The listing builds one solid part. Answer for the finished solid, in the listing's coordinates (mm). Coordinates: 2 decimals unless noted, no trailing zeros. Order: outer loops, then holes, each group sorted by start corner. A loop starts at its lowest first (then second) coordinate and runs counter-clockwise, first axis right, second up. Notation, with made-up numbers: (82, -38) - (133, -38) arc R29 cw to (133, -16) - close; hole circle Ø5 at (-2.75, -4.75). An arc over 180 degrees is marked (long way). Use one line per item in the form item = value. Start each with the question number.
Item 1: Section A-A, the plane z = 0 is taken. Write down the section's boundary in (x, y), and give its area (3 significant figures).
Item 2: The mould has two halves that part along Z. Classify faces 1 (the cylindrical face through (-27.87, 0.76, -8.77)), 2 (the cylindrical face through (-21.9, 0.8, -0.2)), 3 (the flat face through (-28.438, 1, 0)): released by +Z, released by -Z, zero draft, split by the parting line, or undercut.
Item 3: Section B-B, the plane y = 0.8 is taken. Count the separate pieces of the cut face and the enclosed holes in it, and give its area (3 significant figures).
Item 4: This flat-tipped pin is pushed along its axis until it touches: pin 1 Ø1.9 at (x, z) = (-23.44, 0) entering from +Y. Where does it stop, or does it pass through?
Item 5: Consider line 1 along X through (y, z) = (0.6, 0); line 2 along X through (y, z) = (0.25, -0.75); line 3 along Z through (x, y) = (23.5, 1.05) (3 decimals). Determine where each line is inside the solid, lowest interval first. Write a range as [from, to].
from build123d import *

# Parameters (mm, degrees)
SKETCH1_W           = 56.875
SKETCH1_H           = 18.75
BOSS_EXTRUDE1_DEPTH = 1.5
FILLET1_R           = 2
SKETCH2_R           = 1.55
CUT_EXTRUDE1_DEPTH  = 1.5


with BuildPart() as part:
    # Sketch1 → Boss-Extrude1 (new body)
    with BuildSketch(Plane(origin=(0, 0, 0), x_dir=(1, 0, 0), z_dir=(0, 1, 0))):
        Rectangle(SKETCH1_W, SKETCH1_H)
    extrude(amount=BOSS_EXTRUDE1_DEPTH)

    # Fillet1
    fillet1_edges = [part.edges().sort_by_distance(p)[0] for p in [
        (28.4375, 0.75, 9.375),
        (-28.4375, 0.75, 9.375),
        (-28.4375, 0.75, -9.375),
        (28.4375, 0.75, -9.375),
    ]]
    fillet(fillet1_edges, radius=FILLET1_R)

    # Sketch2 → Cut-Extrude1 (cut)
    with BuildSketch(Plane(origin=(0, 1.5, 0), x_dir=(1, 0, 0), z_dir=(0, 1, 0))):
        with Locations(Location((-23.4375, 0, 0), (0, 0, 270))):
            Circle(SKETCH2_R)
        with Locations(Location((23.4375, 0, 0), (0, 0, 270))):
            Circle(SKETCH2_R)
    extrude(amount=-CUT_EXTRUDE1_DEPTH, mode=Mode.SUBTRACT)


solid = part.part
Response:
q1.outline = (-28.44, 0) - (-24.99, 0) - (-24.99, 1.5) - (-28.44, 1.5) - close; (-21.89, 0) - (21.89, 0) - (21.89, 1.5) - (-21.89, 1.5) - close; (24.99, 0) - (28.44, 0) - (28.44, 1.5) - (24.99, 1.5) - close
q1.area = 76.0 mm2
q2.face_1 = released by -Z
q2.face_2 = undercut
q2.face_3 = zero draft
q3.separate_pieces = 1
q3.enclosed_holes = 2
q3.area = 1,050 mm2
q4.pin_1 = through
q5.line_1 = [-28.44, -24.99], [-21.89, 21.89], [24.99, 28.44]
q5.line_2 = [-28.44, -24.79], [-22.08, 22.08], [24.79, 28.44]
q5.line_3 = [-9.375, -1.549], [1.549, 9.375]
